Check sheet for the modelled part. Datum: model origin and axes. Units: mm. A direction names the side the tool comes from. Round coordinates to 2 decimals unless told otherwise and drop trailing zeros. Write each loop counter-clockwise with the first axis right and the second up, starting at its lowest first coordinate (ties: lowest second). Pieces come first, ordered by that corner, then holes. Notation, with made-up numbers: (32.5, -21.5) -> (80.5, -21.5) arc R21 ccw to (80.5, -17.5) -> close; hole circle Ø5 at (-2, -15.5). An arc over 180 degrees is marked (long way). Write item = value, one per line.
Autodesk Inventor part; units mm, degrees
ref_plane "YZ Plane" through (0, 0, 0) normal (1, 0, 0) x (0, 1, 0)
ref_plane "XZ Plane" through (0, 0, 0) normal (0, 1, 0) x (-1, 0, 0)
ref_plane "XY Plane" through (0, 0, 0) normal (0, 0, 1) x (1, 0, 0)
sketch "Sketch1" plane through (0, 0, 0) normal (1, 0, 0) x (0, 1, 0)
  line L0 (-15, -20) -> (15, -20)
  line L1 (15, -20) -> (15, 20)
  line L2 (15, 20) -> (-15, 20)
  line L3 (-15, 20) -> (-15, -20)
  line L4 (-15, -20) -> (15, 20) construction
  line L5 (15, -20) -> (-15, 20) construction
  line L6 (-7, -20) -> (7, -20)
  line L7 (7, -20) -> (7, 20)
  line L8 (7, 20) -> (-7, 20)
  line L9 (-7, 20) -> (-7, -20)
  line L10 (7, -20) -> (5.4606, -20)
  arc A0 (-5.3073, 19.4579) -> (-4.85, 20) centre (-5.4, 20) ccw
  arc A1 (-4.85, 18) -> (-5.3073, 18.5421) centre (-5.4, 18) ccw
  line L11 (-5.4, 20) -> (-5.4, 18) construction
  line L12 (-6, 19.1286) -> (-6, 18.8714)
  line L13 (-5.7921, 19.375) -> (-5.3073, 19.4579)
  line L14 (-5.3073, 18.5421) -> (-5.7921, 18.625)
  arc A2 (-5.7921, 19.375) -> (-6, 19.1286) centre (-5.75, 19.1286) ccw
  arc A3 (-6, 18.8714) -> (-5.7921, 18.625) centre (-5.75, 18.8714) ccw
  line L15 (-5.4, 18) -> (-4.85, 18) construction
  line L16 (-6, 19) -> (-5.4, 19) construction
  line L17 (-4.85, 18) -> (-1.85, 18)
  line L18 (-1.85, 18) -> (-1.85, 20)
  line L19 (7, -20) -> (-7, 20) construction
  line L20 (7, 20) -> (-7, -20) construction
  line L21 (7, 20) -> (15, 20)
  line L22 (15, 20) -> (15, -20)
  line L23 (15, -20) -> (7, -20)
  line L24 (-7, 20) -> (-15, 20)
  line L25 (-15, 20) -> (-15, -20)
  line L26 (-15, -20) -> (-7, -20)
  circle A4 centre (11, 16) radius 2
  circle A5 centre (11, -16) radius 2
  circle A6 centre (-11, 16) radius 2
  circle A7 centre (-11, -16) radius 2
  circle A8 centre (11, -16) radius 3.25
  circle A9 centre (11, 16) radius 3.25
  circle A10 centre (-11, 16) radius 3.25
  circle A11 centre (-11, -16) radius 3.25
  point P0 (0, 0)
  point P1 (0, 0)
  point P2 (5.4606, -20)
  point P3 (11, 20)
  point P4 (-11, 20)
  dimension "d0" = 40
  dimension "d1" = 30
  dimension "d12" = 14
  dimension "d13" = 1.1
  dimension "d14" = 1.6
  dimension "d15" = 1.1
  dimension "d16" = 2
  dimension "d17" = 1
  dimension "d18" = 0.25
  dimension "d19" = 0.75
  dimension "d20" = 3
  dimension "d21" = 40
  dimension "d22" = 30
  dimension "d23" = 4
  dimension "d24" = 4
  dimension "d25" = 4
  dimension "d26" = 4
  dimension "d27" = 4
  dimension "d28" = 4
  dimension "d29" = 4
  dimension "d30" = 4
  dimension "d31" = 4
  dimension "d32" = 4
  dimension "d33" = 4
  dimension "d34" = 4
  dimension "d37" = 6.5
  dimension "d38" = 6.5
  dimension "d39" = 6.5
  dimension "d40" = 6.5
extrude "Extrusion1" add sketch "Sketch1" along normal blind 14 contours L3 L2 L9 L0 | L9 L2 A0 L13 A2 L12 A3 L14 A1 L17 L18 L7 L0 | L7 L2 L1 L0 | L2 L18 L17 A1 L14 A3 L12 A2 L13 A0 | A4 | A5 | A6 | A7 | A8 | A9 | A10 | A11
sketch "Sketch2" plane through (0, 15, 20) normal (0, 1, 0) x (1, 0, 0)
  line L0 (0, 40) -> (0, 0) construction
  line L1 (0, 11) -> (5, 11) construction
  line L2 (0, 29) -> (5, 29) construction
  circle A0 centre (5, 11) radius 2
  circle A1 centre (5, 29) radius 2
  line L3 (0, 0) -> (14, 0)
  point P0 (0, 20)
  dimension "d4" = 5
  dimension "d5" = 5
  dimension "d6" = 4
  dimension "d7" = 4
  dimension "d8" = 18
  dimension "d9" = 11
extrude "Extrusion2" cut sketch "Sketch2" against normal blind 3
mirror "Mirror1" about plane through (0, 0, 0) normal (0, 1, 0) of "Extrusion2"
extrude "Extrusion3" cut sketch "Sketch1" along normal through all contours A4 | A5 | A6 | A7
extrude "Extrusion4" cut sketch "Sketch1" along normal blind 5 contours A8 | A9 | A10 | A11
equation "\"d27\" = d26"
equation "\"d30\" = d27"
equation "\"d31\" = d25"
equation "\"d32\" = d23"
equation "\"d34\" = d23"
equation "\"d38\" = d37"
equation "\"d39\" = d37"
equation "\"d40\" = d37"
equation "\"d5\" = d4"
properties part number "LRT_Face"
(1) Sectioned sample at C-C on x = 2.5. Enter the section's corners in (y, z).
Worked answers:
outline = (-15, -20) -> (15, -20) -> (15, 20) -> (-15, 20) -> close; hole circle Ø6.5 at (-11, -16); hole circle Ø6.5 at (-11, 16); hole circle Ø6.5 at (11, -16); hole circle Ø6.5 at (11, 16)
(2) Release check for a two-part mould opening along X. For faces 1 (the cylindrical face through (9, -11, 14)), 2 (the flat face through (5, -12, -9)), 3 (the flat face through (5, 13, 15)), 4 (the flat face through (5, 12, 9)) record: pulls with the +X half, pulls with the -X half, needs draft (parallel to the pull), parting line crosses it, or undercut.
Worked answers:
face_1 = needs draft
face_2 = undercut
face_3 = pulls with the -X half
face_4 = undercut
(3) Material ranges on L1, parallel to Z at x = 1, y = 11; L2, parallel to Y at x = 9.25, z = -16; L3, parallel to X at y = -13.65, z = -9, recorded low to high. Write a range as [from, to].
Worked answers:
L1 = [-20, -19.25], [-12.75, 12.75], [19.25, 20]
L2 = [-15, -13], [-9, 9], [13, 15]
L3 = [0, 3], [7, 14]
(4) Sectioned sample at B-B on y = 11. Enter the section's corners in (x, z), then the cut area to 3 significant figures.
Worked answers:
outline = (0, -20) -> (14, -20) -> (14, -18) -> (5, -18) -> (5, -19.25) -> (0, -19.25) -> close; (0, -12.75) -> (5, -12.75) -> (5, -14) -> (14, -14) -> (14, 14) -> (5, 14) -> (5, 12.75) -> (0, 12.75) -> close; (0, 19.25) -> (5, 19.25) -> (5, 18) -> (14, 18) -> (14, 20) -> (0, 20) -> close
area = 423 mm²
(5) Sectioned sample at D-D on z = -9. Enter the section's corners in (x, y), then the cut area to 3 significant figures.
Worked answers:
outline = (0, -15) -> (3, -15) -> (3, -12) -> (7, -12) -> (7, -15) -> (14, -15) -> (14, 15) -> (7, 15) -> (7, 12) -> (3, 12) -> (3, 15) -> (0, 15) -> close
area = 396 mm²
(6) Access from +Z, -Z, +X, -X, +Y, -Y to the whole of each face (thin tool, end or side, straight path). Record for faces 5 (the flat face through (7, 15, 0)), 6 (the flat face through (5, -9, 15)), 7 (the cylindrical face through (3.526, -13.521, -7.648)), 8 (the flat face through (7, 0, -20)), 9 (the cylindrical face through (3.526, 13.521, 7.648)).
Worked answers:
face_5 = +Z, -Z, +X, -X, +Y
face_6 = -X
face_7 = -Y
face_8 = -Z, +X, -X, +Y, -Y
face_9 = +Y
(7) Go/stop test with flat-tipped pins: P1, Ø6, axis at y = 11, z = -16, coming from the -X side; P2, Ø7.5, axis at y = -11, z = 16, coming from the -X side; P3, Ø2, axis at x = 4.5, z = 9, coming from the +Y side; P4, Ø3, axis at x = 5, z = 9, coming from the -Y side. Record where each tip stops, or that it passes through.
Worked answers:
P1 = 5
P2 = 0
P3 = 12
P4 = -12
(8) Sectioned sample at A-A on z = -16. Enter the section's corners in (x, y), then the cut area to 3 significant figures.
Worked answers:
outline = (0, -15) -> (14, -15) -> (14, -13) -> (5, -13) -> (5, -14.25) -> (0, -14.25) -> close; (0, -7.75) -> (5, -7.75) -> (5, -9) -> (14, -9) -> (14, 9) -> (5, 9) -> (5, 7.75) -> (0, 7.75) -> close; (0, 14.25) -> (5, 14.25) -> (5, 13) -> (14, 13) -> (14, 15) -> (0, 15) -> close
area = 283 mm²
